Can you work these out from the model? Positions are in its coordinate system, mm. A direction names the side the tool comes from. Give positions to 0.01 mm unless a question says otherwise; leave off trailing zeros. Order: outer loops, then holes, each group sorted by start corner. A loop starts at its lowest first (then second) coordinate and runs counter-clockwise, first axis right, second up. Notation, with made-up numbers: M 36,38.25 L 65,38.25 A10 ccw 65,55.25 Z; hole C -37.75,-18 d7. An arc over 180 degrees is marked long. Write each question's results on one line, items separated by ' | '.
from build123d import *

# Parameters (mm, degrees)
SKETCH065_R             = 17.25
SKETCH065_R_2           = 2.75
SKETCH065_R_3           = 1.7
PAD030_DEPTH            = 5
SKETCH066_R             = 2.7
POCKET034_DEPTH         = 101.092794
POLARPATTERN006_COUNT   = 2
SKETCH068_R             = 0.75
POCKET035_DEPTH         = 17.251
POCKET035_DEPTH_BACK    = 17.251
SKETCH078_R             = 10.15
POCKET045_DEPTH         = 2.5
POCKET046_DEPTH         = 103.092794
BODY017_PLACEMENT_ANGLE = 270


with BuildPart() as part:
    # Sketch065 → Pad030 (new body)
    with BuildSketch(Plane.XZ):
        Circle(SKETCH065_R)
        Circle(SKETCH065_R_2, mode=Mode.SUBTRACT)
        with Locations((0, 7)):
            Circle(SKETCH065_R_3, mode=Mode.SUBTRACT)
        with Locations((-7, 0)):
            Circle(SKETCH065_R_3, mode=Mode.SUBTRACT)
        with Locations((0, -7)):
            Circle(SKETCH065_R_3, mode=Mode.SUBTRACT)
        with Locations((7, 0)):
            Circle(SKETCH065_R_3, mode=Mode.SUBTRACT)
    extrude(amount=PAD030_DEPTH)

    # Sketch066 → Pocket034 (cut, through all)
    with BuildSketch(Plane.XZ.offset(2)):
        with Locations((0, 7)):
            Circle(SKETCH066_R)
    pocket034 = extrude(amount=POCKET034_DEPTH, mode=Mode.SUBTRACT)

    # PolarPattern006: Pocket034 ×2 about axis
    polarpattern006_axis = Axis((0, -2, 0), (0, -1, 0))
    for i in range(1, POLARPATTERN006_COUNT):
        add(pocket034.rotate(polarpattern006_axis, i * 360 / POLARPATTERN006_COUNT), mode=Mode.SUBTRACT)

    # Sketch067 → Groove004 (revolve, cut)
    with BuildSketch(Plane.YZ):
        with BuildLine():
            ThreePointArc((-4, 17.25), (-2.5, 15.75), (-1, 17.25))
            Line((-4, 17.25), (-1, 17.25))
        make_face()
    revolve(axis=Axis((0, 0, 0), (0, 1, 0)), mode=Mode.SUBTRACT)

    # Sketch068 → Pocket035 (cut, two sides)
    with BuildSketch(Plane.XY) as pocket035_sk:
        with Locations((0, -3)):
            Circle(SKETCH068_R)
    extrude(amount=-POCKET035_DEPTH, mode=Mode.SUBTRACT)
    extrude(pocket035_sk.sketch, amount=POCKET035_DEPTH_BACK, mode=Mode.SUBTRACT)

    # Sketch078 → Pocket045 (cut)
    with BuildSketch(Plane.XZ):
        Circle(SKETCH078_R)
    extrude(amount=POCKET045_DEPTH, mode=Mode.SUBTRACT)

    # Sketch080 → Pocket046 (cut, through all)
    with BuildSketch(Plane.XZ):
        with BuildLine():
            ThreePointArc((-0.5, 4.146692), (4e-06, 3.646692), (0.5, 4.1467))
            Line((0.5, 4.1467), (0.5, 4.3467))
            Line((0.5, 4.3467), (-0.5, 4.3467))
            Line((-0.5, 4.3467), (-0.5, 4.146692))
        make_face()
    pocket046 = extrude(amount=POCKET046_DEPTH, mode=Mode.SUBTRACT)

    # Mirrored008: Pocket046 across Sketch080 H_Axis
    add(pocket046.mirror(Plane(origin=(0, 0, 0), x_dir=(0, -1, 0), z_dir=(0, 0, 1))), mode=Mode.SUBTRACT)


with BuildPart() as part_1:
    # Body017 placement: moved
    add(part.part.moved(Location((0, 0, 2.5))).rotate(Axis((0, 0, 2.5), (1, 0, 0)), BODY017_PLACEMENT_ANGLE))


solid = part_1.part
(1) Will these pins go through, and if not, where does the flat tip stop? P1, Ø7, axis at x = 0, y = 0, coming from the -Z side; P2, Ø3, axis at x = -7.5, z = 3.5, coming from the -Y side; P3, Ø2, axis at y = 10.5, z = 3.5, coming from the +X side; P4, Ø0.9, axis at x = 0, z = 5.5, coming from the -Y side.
Data:
P1: stops at z = 5 | P2: stops at y = -16.17 | P3: stops at x = 14.4 | P4: passes through
(2) I need wall thicknesses on L1, parallel to Z at x = 10.5, y = -13.5; L2, parallel to Z at x = 0, y = -12; L3, parallel to Z at x = 10, y = 1.5. Which ranges of each line are inside material? Lowest first, please. Write a range as from..to.
Data:
L1: z = 2.5..3.51, 6.49..7.5 | L2: z = 2.5..4.75, 6.25..7.5 | L3: z = 5..7.5
(3) We'd pull the mould along Z, two halves only. Please class faces 1 (the face through (5.3, 0.07, 6.23)), 2 (the face through (-0.02, 3.32, 6.25)), 3 (the face through (-4, 0, 5)), 4 (the face through (-0.02, -3.32, 6.25)): +Z half, -Z half, draft (parallel to the pull), parting line (faces both ways), or undercut.
Data:
face 1: draft | face 2: undercut | face 3: -Z half | face 4: undercut
(4) Imagine slicing it at C-C, the plane z = 2.95. Write out the boundary of the cut face in (x, y), plus the area to 3 significant figures.
Data:
outline: C 0,0 d34.5; hole C 0,0 d20.3 | area: 611 mm2
(5) Imagine slicing it at B-B, the plane x = 0. Write out the boundary of the cut face in (y, z).
Data:
outline: M -17.25,2.5 L -10.15,2.5 L -10.15,4.75 L -15.77,4.75 A1.5 cw -17.25,3.5 Z; M -17.25,6.5 A1.5 cw -16.42,6.25 L -9.7,6.25 L -9.7,7.5 L -17.25,7.5 Z; M -3.65,6.25 L -2.75,6.25 L -2.75,7.5 L -3.65,7.5 Z; M 2.75,6.25 L 3.65,6.25 L 3.65,7.5 L 2.75,7.5 Z; M 9.7,6.25 L 16.42,6.25 A1.5 cw 17.25,6.5 L 17.25,7.5 L 9.7,7.5 Z; M 10.15,2.5 L 17.25,2.5 L 17.25,3.5 A1.5 cw 15.77,4.75 L 10.15,4.75 Z
(6) For faces 5 (the face through (-8.05, -6.18, 3.73)), 6 (the face through (7.4, -7.4, 2.5)), 7 (the face through (-0.011, 3.647, 6.769)), which set-ups out of +Z, -Z, +X, -X, +Y, -Y let a thin tool reach every point of the face, with its end or its side?
Data:
face 5: -Z | face 6: -Z, +X, -X, +Y, -Y | face 7: +Z, -Z
(7) Imagine slicing it at A-A, the plane z = 5.5. Write out the boundary of the cut face in (x, y), plus the area to 3 significant figures.
Data:
outline: M -0.75,-15.82 L -0.75,-9.59 A2.7 cw -0.75,-4.41 L -0.75,-2.65 A2.75 cw -0.75,2.65 L -0.75,4.41 A2.7 cw -0.75,9.59 L -0.75,15.82 A15.84 ccw Z; M 0.75,-15.82 A15.84 ccw 0.75,15.82 L 0.75,9.59 A2.7 cw 0.75,4.41 L 0.75,2.65 A2.75 cw 0.75,-2.65 L 0.75,-4.41 A2.7 cw 0.75,-9.59 Z; hole C -7,0 d3.4; hole C 7,0 d3.4 | area: 677 mm2
